```python
from build123d import *

# Parameters (mm, degrees)
BOSS_EXTRUDE1_DEPTH  = 3
SKETCH3_W            = 18
SKETCH3_H            = 6
BOSS_EXTRUDE2_DEPTH  = 2
SKETCH4_R            = 1.5
CUT_EXTRUDE1_DEPTH   = 14
FILLET1_R            = 1
SKETCH5_W            = 3.3
SKETCH5_H            = 5.2
CUT_EXTRUDE2_DEPTH   = 0.25
SKETCH6_W            = 0.5
SKETCH6_H            = 3
CUT_EXTRUDE3_DEPTH   = 0.35
SKETCH7_W            = 12
SKETCH7_H            = 5
CUT_EXTRUDE4_DEPTH   = 2
SKETCH8_W            = 0.3
SKETCH8_H            = 0.3
BOSS_EXTRUDE3_DEPTH  = 12
LPATTERN1_COUNT      = 2
LPATTERN1_PITCH      = 9
LPATTERN1_COUNT_DIR2 = 2
LPATTERN1_PITCH_DIR2 = 2.5


with BuildPart() as part:
    # Sketch1 → Boss-Extrude1 (new body, symmetric)
    with BuildSketch(Plane.XY):
        Polygon((-9, 12.1), (-13, 12.1), (-13, 0), (0, 0), (0, 12.1), (-4, 12.1), (-4, 3), (-9, 3), align=None)
    extrude(amount=BOSS_EXTRUDE1_DEPTH, both=True)

    # Sketch3 → Boss-Extrude2 (add)
    with BuildSketch(Plane.ZY.offset(13)):
        with Locations((0, 3)):
            Rectangle(SKETCH3_W, SKETCH3_H)
    extrude(amount=-BOSS_EXTRUDE2_DEPTH)

    # Sketch4 → Cut-Extrude1 (cut, through all)
    with BuildSketch(Plane.ZY.offset(13)):
        with Locations((-5.5, 3)):
            Circle(SKETCH4_R)
        with Locations((5.5, 3)):
            Circle(SKETCH4_R)
    extrude(amount=-CUT_EXTRUDE1_DEPTH, mode=Mode.SUBTRACT)

    # Fillet1
    fillet1_edges = [part.edges().sort_by_distance(p)[0] for p in [
        (-12, 6, -9),
        (-12, 0, -9),
        (-12, 6, 9),
        (-12, 0, 9),
    ]]
    fillet(fillet1_edges, radius=FILLET1_R)

    # Sketch5 → Cut-Extrude2 (cut)
    with BuildSketch(Plane(origin=(0, 12.1, 0), x_dir=(1, 0, 0), z_dir=(0, 1, 0))):
        with Locations((-11, 0)):
            Rectangle(SKETCH5_W, SKETCH5_H)
    cut_extrude2 = extrude(amount=-CUT_EXTRUDE2_DEPTH, mode=Mode.SUBTRACT)

    # Sketch6 → Cut-Extrude3 (cut)
    with BuildSketch(Plane(origin=(-9, 0, 0), x_dir=(0, 0, -1), z_dir=(1, 0, 0))):
        with Locations((0, 10.6)):
            Rectangle(SKETCH6_W, SKETCH6_H)
    cut_extrude3 = extrude(amount=-CUT_EXTRUDE3_DEPTH, mode=Mode.SUBTRACT)

    # Mirror1: Cut-Extrude2, Cut-Extrude3 across plane
    add(cut_extrude2.mirror(Plane(origin=(-6.5, 0, 0), x_dir=(0, 0, 1), z_dir=(1, 0, 0))), mode=Mode.SUBTRACT)
    add(cut_extrude3.mirror(Plane(origin=(-6.5, 0, 0), x_dir=(0, 0, 1), z_dir=(1, 0, 0))), mode=Mode.SUBTRACT)

    # Sketch7 → Cut-Extrude4 (cut)
    with BuildSketch(Plane.XZ):
        with Locations((-6.5, 0)):
            Rectangle(SKETCH7_W, SKETCH7_H)
    extrude(amount=-CUT_EXTRUDE4_DEPTH, mode=Mode.SUBTRACT)

    # Sketch8 → Boss-Extrude3 (add)
    with BuildSketch(Plane.XZ.offset(-2)):
        with Locations((-11, 1.25)):
            Rectangle(SKETCH8_W, SKETCH8_H)
    boss_extrude3 = extrude(amount=BOSS_EXTRUDE3_DEPTH)

    # LPattern1: Boss-Extrude3 2 × 2
    with Locations(*[(i * LPATTERN1_PITCH, 0, -j * LPATTERN1_PITCH_DIR2) for i in range(LPATTERN1_COUNT) for j in range(LPATTERN1_COUNT_DIR2) if (i, j) != (0, 0)]):
        add(boss_extrude3)


solid = part.part
```
Work out the finished part from the listing and answer in its coordinate system (mm). A direction names the side the tool comes from. Coordinates: 2 decimals unless noted, no trailing zeros. Loops run counter-clockwise (first coordinate to the right, second up) from the corner with the lowest first, then second, coordinate; pieces in that order, holes last.
1) For a pull along Z with two mould halves and no side action, classify faces 5 (the flat face through (-6, 3, 0)), 6 (the cylindrical face through (-12, 2.1, 4.3)), 7 (the cylindrical face through (-11.986, 5.699, -8.715)), 8 (the flat face through (-7, 1, -2.5)) as +Z half, -Z half, draft (parallel to the pull), parting line (faces both ways), or undercut.
Results:
face 5: draft
face 6: undercut
face 7: -Z half
face 8: undercut
2) Section B-B (y = -7.75) is taken. Give the vertices of the cut face in (x, z).
Results:
outline: (-11.15, -1.4) - (-10.85, -1.4) - (-10.85, -1.1) - (-11.15, -1.1) - close; (-11.15, 1.1) - (-10.85, 1.1) - (-10.85, 1.4) - (-11.15, 1.4) - close; (-2.15, -1.4) - (-1.85, -1.4) - (-1.85, -1.1) - (-2.15, -1.1) - close; (-2.15, 1.1) - (-1.85, 1.1) - (-1.85, 1.4) - (-2.15, 1.4) - close
3) For faces 1 (the flat face through (-11, 3, 7.3)), 2 (the flat face through (-12.5, 1, 0)), 3 (the flat face through (-12, 6, 5)), 4 (the flat face through (-12, 6, -6)), determine the directions among +Z, -Z, +X, -X, +Y, -Y from which every point of the face is accessible in a straight line to the end or side of a thin tool.
Results:
face 1: +Z, +X, +Y, -Y
face 2: -Y
face 3: +Z, +X, -X, +Y
face 4: -Z, +X, -X, +Y
4) Section C-C (y = 7) is taken. Give the vertices of the cut face in (x, z).
Results:
outline: (-13, -3) - (-9, -3) - (-9, 3) - (-13, 3) - close; (-4, -3) - (0, -3) - (0, 3) - (-4, 3) - close
5) Consider probe 1 along X at (y, z) = (8.5, -0.5); probe 2 along Y at (x, z) = (-11.75, 5.5); probe 3 along Y at (x, z) = (-8, 2.75). Determine where each line is inside the solid, lowest interval first.
Results:
probe 1: x = -13 to -9, -4 to 0
probe 2: y = 0 to 1.5, 4.5 to 6
probe 3: y = 0 to 3
6) Section A-A (z = -5.5) is taken. Give the vertices of the cut face in (x, y), plus the area to 3 significant figures.
Results:
outline: (-13, 0) - (-11, 0) - (-11, 1.5) - (-13, 1.5) - close; (-13, 4.5) - (-11, 4.5) - (-11, 6) - (-13, 6) - close
area: 6.00 mm2
7) Section D-D (z = -0.75) is taken. Give the vertices of the cut face in (x, y), plus the area to 4 significant figures.
Results:
outline: (-13, 0) - (-12.5, 0) - (-12.5, 2) - (-0.5, 2) - (-0.5, 0) - (0, 0) - (0, 12.1) - (-0.35, 12.1) - (-0.35, 11.85) - (-3.65, 11.85) - (-3.65, 12.1) - (-4, 12.1) - (-4, 3) - (-9, 3) - (-9, 12.1) - (-9.35, 12.1) - (-9.35, 11.85) - (-12.65, 11.85) - (-12.65, 12.1) - (-13, 12.1) - close
area: 86.15 mm2
8) Flat-ended cylindrical pins translate along their axes: pin 1 (2 mm diameter, centred on x = -2, y = 3.5, fed in from -Z); pin 2 (1.5 mm diameter, centred on x = -4, z = -5, fed in from -Y); pin 3 (6 mm diameter, centred on x = -11, y = -0.5, fed in from +Z); pin 4 (1.6 mm diameter, centred on x = -8, y = 0.5, fed in from +Z). Find the tip coordinate at first contact, or state that the pin passes through.
Results:
pin 1: stops at z = -3
pin 2: passes through
pin 3: stops at z = 9
pin 4: stops at z = 3
